from build123d import *

# Parameters (mm, degrees)
SKETCH1_W           = 91.2368
SKETCH1_H           = 66.8782
BASE_FLANGE1_DEPTH  = 0.7366
SKETCH6_W           = 91.2368
SKETCH6_H           = 66.8782
BOSS_EXTRUDE1_DEPTH = 37.7952
SKETCH8_W           = 8.763
SKETCH8_H           = 66.8782
CUT_EXTRUDE2_DEPTH  = 18.8976
FILLET1_R           = 10.16


# Sheet-metal steps are written as plain solids
with BuildPart() as part:
    # Sketch1 → Base-Flange1 (new body)
    with BuildSketch(Plane.XY):
        with Locations((0, 33.4391)):
            Rectangle(SKETCH1_W, SKETCH1_H)
    extrude(amount=-BASE_FLANGE1_DEPTH)

    # Sketch6 → Boss-Extrude1 (add)
    with BuildSketch(Plane.XY):
        with Locations((0, 33.4391)):
            Rectangle(SKETCH6_W, SKETCH6_H)
    extrude(amount=BOSS_EXTRUDE1_DEPTH)

    # Sketch8 → Cut-Extrude2 (cut)
    with BuildSketch(Plane.XY.offset(37.7952)):
        with Locations((-41.2369, 33.4391)):
            Rectangle(SKETCH8_W, SKETCH8_H)
    cut_extrude2 = extrude(amount=-CUT_EXTRUDE2_DEPTH, mode=Mode.SUBTRACT)

    # Mirror1: Cut-Extrude2 across plane
    add(cut_extrude2.mirror(Plane(origin=(0, 0, 0), x_dir=(0, 0, 1), z_dir=(1, 0, 0))), mode=Mode.SUBTRACT)

    # Fillet1
    # the kernel refuses this fillet: 10.16 mm, written as the material it takes off along each edge
    with BuildSketch(Plane(origin=(-45.6184, -25.158744876, 18.8976), x_dir=(1, 0, 0), z_dir=(0, 1, 0))) as fillet1_piece_1:
        with BuildLine():
            CenterArc((10.16, 10.063497951), FILLET1_R, 180, 82.096792267)
            Line((0, 10.063497951), (-0.2032, 10.063497951))
            Line((-0.2032, 10.063497951), (-0.2032, 0))
            Line((-0.2032, 0), (0, -0.2032))
            ThreePointArc((0, -0.2032), (4.3815, -0.2032), (8.73506, -0.201269959))
            Line((8.73506, -0.201269959), (8.763, 0))
        make_face()
    extrude(amount=117.195689753, mode=Mode.SUBTRACT)
    with BuildSketch(Plane(origin=(45.6184, -25.158744876, 18.8976), x_dir=(-1, 0, 0), z_dir=(0, 1, 0))) as fillet1_piece_2:
        with BuildLine():
            CenterArc((10.16, -10.063497951), FILLET1_R, 97.903207733, 82.096792267)
            Line((0, -10.063497951), (-0.2032, -10.063497951))
            Line((-0.2032, -10.063497951), (-0.2032, 0))
            Line((-0.2032, 0), (0, 0.2032))
            ThreePointArc((0, 0.2032), (4.3815, 0.2032), (8.73506, 0.201269959))
            Line((8.73506, 0.201269959), (8.763, 0))
        make_face()
    extrude(amount=117.195689753, mode=Mode.SUBTRACT)
    with BuildSketch(Plane(origin=(36.8554, 92.2782, 37.7952), x_dir=(-1, 0, 0), z_dir=(0, -1, 0)), Plane(origin=(-36.8554, 92.2782, 37.7952), x_dir=(0, 0, -1), z_dir=(0, -1, 0)), Plane(origin=(-45.6184, 92.2782, -0.7366), x_dir=(1, 0, 0), z_dir=(0, -1, 0))) as fillet1_piece_3:
        with BuildLine():
            CenterArc((FILLET1_R, FILLET1_R), FILLET1_R, 180, 90)
            Line((0, FILLET1_R), (-FILLET1_R * 0.02, FILLET1_R))
            Line((-FILLET1_R * 0.02, FILLET1_R), (-FILLET1_R * 0.02, -FILLET1_R * 0.02))
            Line((-FILLET1_R * 0.02, -FILLET1_R * 0.02), (FILLET1_R, -FILLET1_R * 0.02))
            Line((FILLET1_R, -FILLET1_R * 0.02), (FILLET1_R, 0))
        make_face()
    extrude(amount=117.6782, mode=Mode.SUBTRACT)
    with BuildSketch(Plane(origin=(45.6184, -25.4, -0.7366), x_dir=(0, 0, 1), z_dir=(0, 1, 0))) as fillet1_piece_4:
        with BuildLine():
            CenterArc((FILLET1_R, -FILLET1_R), FILLET1_R, 90, 90)
            Line((0, -FILLET1_R), (-FILLET1_R * 0.02, -FILLET1_R))
            Line((-FILLET1_R * 0.02, -FILLET1_R), (-FILLET1_R * 0.02, FILLET1_R * 0.02))
            Line((-FILLET1_R * 0.02, FILLET1_R * 0.02), (FILLET1_R, FILLET1_R * 0.02))
            Line((FILLET1_R, FILLET1_R * 0.02), (FILLET1_R, 0))
        make_face()
    extrude(amount=117.6782, mode=Mode.SUBTRACT)


solid = part.part
Can you work these out from the model? Positions are in its coordinate system, mm. A direction names the side the tool comes from. Give positions to 0.01 mm unless a question says otherwise; leave off trailing zeros. Write each loop counter-clockwise with the first axis right and the second up, starting at its lowest first coordinate (ties: lowest second). Pieces come first, ordered by that corner, then holes. Notation, with made-up numbers: M 66,61 L 71,61 A33 ccw 71,91 Z; hole C -14.75,25.5 d6. An arc over 180 degrees is marked long. Answer in a Markdown table with one row per item. Add a question column.
Item 1: Imagine slicing it at A-A, the plane y = 8.5. Write out the boundary of the cut face in (x, z), plus the area to 3 significant figures.
Item 2: Imagine slicing it at B-B, the plane z = 15. Write out the boundary of the cut face in (x, y).
Item 3: We'd pull the mould along Y, two halves only. Please class faces 4 (the flat face through (0, 34, 37.795)), 5 (the flat face through (-1, 66.878, 18)), 6 (the flat face through (-1, 0, 18)): released by +Y, released by -Y, zero draft, split by the parting line, or undercut.
Item 4: For pin 1 Ø4 at (y, z) = (7, 21) entering from -X; pin 2 Ø4.5 at (y, z) = (42.5, 23.5) entering from +X, each with a flat end and sliding along its axis, tell me the tip position at first contact or that it passes through.
Item 5: On a 3-axis mill with a long thin cutter (end or side, diameter ignored), from which of +Z, -Z, +X, -X, +Y, -Y can I reach the whole of each face in a straight line? I mean faces 1 (the cylindrical face through (42.616, 32.971, 2.213)), 2 (the flat face through (36.855, 33, 23)), 3 (the flat face through (-36.855, 33, 23)). Say none if no direction works.
Item 6: Imagine slicing it at C-C, the plane z = 31. Write out the boundary of the cut face in (x, y).
Item 7: Please list where these lines run through material, in increasing order: L1, parallel to X at y = 53, z = 23; L2, parallel to Z at x = 34, y = 63; L3, parallel to X at y = 20, z = 32.
Evaluation:
| question | item | result |
|---|---|---|
| 1 | outline | M -45.61,9.13 A10.16 ccw -35.46,-0.74 L 35.46,-0.74 A10.16 ccw 45.61,9.13 A10.16 ccw 36.86,18.9 L 36.86,27.64 A10.16 ccw 26.7,37.8 L -26.7,37.8 A10.16 ccw -36.86,27.64 L -36.86,18.9 A10.16 ccw Z |
| 1 | area | 3,050 mm² |
| 2 | outline | M -43.53,0 L 43.53,0 L 43.53,66.88 L -43.53,66.88 Z |
| 3 | face 4 | zero draft |
| 3 | face 5 | released by +Y |
| 3 | face 6 | released by -Y |
| 4 | pin 1 | stops at x = -36.86 |
| 4 | pin 2 | stops at x = 36.86 |
| 5 | face 1 | -Z, +X, +Y, -Y |
| 5 | face 2 | +Z, +X, +Y, -Y |
| 5 | face 3 | +Z, -X, +Y, -Y |
| 6 | outline | M -36.28,0 L 36.28,0 L 36.28,66.88 L -36.28,66.88 Z |
| 7 | L1 | x = -36.86 to 36.86 |
| 7 | L2 | z = -0.74 to 34.7 |
| 7 | L3 | x = -35.87 to 35.87 |
